Source: CAD feature listing. Evaluate the final solid. Frame: model axes, mm. A direction names the side the tool comes from. Give positions to 0.01 mm unless a question says otherwise; leave off trailing zeros. Order: outer loops, then holes, each group sorted by start corner. A loop starts at its lowest first (then second) coordinate and runs counter-clockwise, first axis right, second up. Notation, with made-up numbers: (70.25, 57) - (91.25, 57) arc R33 ccw to (91.25, 87) - close; hole circle Ø11 at (24, -32.5). An arc over 180 degrees is marked (long way). Use CSV: the item, a comma, the result in double quotes.
```python
from build123d import *
from build123d.topology import SkipClean

# Parameters (mm, degrees)
SKETCH1_3_W              = 17.39
SKETCH1_3_H              = 14
REVOLVE2_ANGLE           = 3
REVOLVE2_OTHER_WAY_ANGLE = 3
CIRPATTERN1_COUNT        = 6
CIRPATTERN1_ANGLE        = 25


with BuildPart() as part:
    # Sketch1 → Revolve1 (revolve)
    with BuildSketch(Plane.YZ, mode=Mode.PRIVATE) as revolve1_sk:
        Polygon((120, 13), (13, 13), (13, 4), (10, 4), (10, 3), (0, 3), (0, 0), (19, 0), (19, 10), (129, 10), (129, -5), (152.39, -5), (152.39, 5), (135, 5), (135, 19), (120, 19), align=None)
    revolve(revolve1_sk.sketch.rotate(Axis((0, 0, 0), (0, 0, 1)), 90), axis=Axis((0, 0, 0), (0, 0, 1)))

    # Sketch1<3> → Revolve2 (revolve)
    with BuildSketch(Plane.YZ):
        with Locations((143.695, 12)):
            Rectangle(SKETCH1_3_W, SKETCH1_3_H)
    revolve(axis=Axis((0, 0, 0), (0, 0, 1)), revolution_arc=REVOLVE2_ANGLE)

    # Sketch1<3> → Revolve2 other way (revolve)
    with SkipClean():  # the faces are left unmerged after this step: merging them gives an invalid solid
        with BuildSketch(Plane.YZ):
            with Locations((143.695, 12)):
                Rectangle(SKETCH1_3_W, SKETCH1_3_H)
        revolve(axis=Axis((0, 0, 0), (0, 0, -1)), revolution_arc=REVOLVE2_OTHER_WAY_ANGLE)
    add(part.part.scale(1), mode=Mode.REPLACE)  # the faces are merged on a copy

    # Sketch2 → Cut-Revolve4 (revolve, cut)
    with BuildSketch(Plane(origin=(0, 0, 8), x_dir=(0, 1, 0), z_dir=(0, 0, 1)), mode=Mode.PRIVATE) as cut_revolve4_sk:
        Polygon((111.823962377, 11.376893011), (151.671750301, 14.863122721), (151.810110042, 13.281663637), (111.962322119, 9.795433927), align=None)
    cut_revolve4 = revolve(cut_revolve4_sk.sketch.rotate(Axis((-9.795433927, 111.962322119, 8), (-0.08715574274765829, 0.9961946980917455, 0)), 180), axis=Axis((-9.795433927, 111.962322119, 8), (-0.08715574274765829, 0.9961946980917455, 0)), mode=Mode.SUBTRACT)

    # CirPattern1: Cut-Revolve4 ×6 about axis
    cirpattern1_axis = Axis((0, 0, 0), (0, 0, 1))
    for i in range(1, CIRPATTERN1_COUNT):
        add(cut_revolve4.rotate(cirpattern1_axis, i * CIRPATTERN1_ANGLE / (CIRPATTERN1_COUNT - 1)), mode=Mode.SUBTRACT)


solid = part.part
```
Item 1: First-contact query: pin 1 (6 mm diameter, centred on y = -119, z = -1.5, fed in from +X); pin 2 (10 mm diameter, centred on x = -75, z = 7.5, fed in from +Y); pin 3 (16 mm diameter, centred on x = -4, y = 2, fed in from +Z). Flat tips, straight axial feed; report the tip coordinate or a pass-through.
Filled in:
pin 1,"stops at x = 98.83"
pin 2,"stops at y = 135.01"
pin 3,"stops at z = 4"
Item 2: Mould query, pull axis X, two halves, no side actions, for faces 5 (the flat face through (-7.514, 143.377, 12.098)), 6 (the cylindrical face through (4.119, 18.548, 5.07)), 7 (the flat face through (1, -136, 5)). Classes: released by +X, released by -X, zero draft, split by the parting line, or undercut.
Filled in:
face 5,"released by -X"
face 6,"undercut"
face 7,"zero draft"
Item 3: Material intervals for line 1 (Y direction, x = 0, z = 3.6); line 2 (Y direction, x = 0, z = 5.25); line 3 (Y direction, x = 0, z = 10.5), sorted ascending. Write a range as from..to.
Filled in:
line 1,"y = -152.39..-129, -19..-10, 10..19, 129..152.39"
line 2,"y = -135..-129, -19..-13, 13..19, 129..152.39"
line 3,"y = -135..-13, 13..152.39"
Item 4: Section B-B on x = -113. Return the cut outline in (y, z), then the cut area to 3 significant figures.
Filled in:
outline,"(-102.24, -5) - (-62.23, -5) - (-62.23, 10) - (62.23, 10) - (62.23, -5) - (102.24, -5) - (102.24, 5) - (73.86, 5) - (73.86, 19) - (40.39, 19) - (40.39, 13) - (-40.39, 13) - (-40.39, 19) - (-73.86, 19) - (-73.86, 5) - (-102.24, 5) - close"
area,"1,760 mm2"
Item 5: Section A-A on y = -30.5. Return the cut outline in (x, z), then the cut area to 3 significant figures.
Filled in:
outline,"(-149.31, -5) - (-125.34, -5) - (-125.34, 10) - (125.34, 10) - (125.34, -5) - (149.31, -5) - (149.31, 5) - (131.51, 5) - (131.51, 19) - (116.06, 19) - (116.06, 13) - (-116.06, 13) - (-116.06, 19) - (-131.51, 19) - (-131.51, 5) - (-149.31, 5) - close"
area,"1,520 mm2"
Item 6: Set-up query: faces 1 (the cylindrical face through (10.316, 7.91, 8.437)), 2 (the flat face through (7.514, 143.377, 12.098)), 3 (the flat face through (-125, -35, -5)), 4 (the cylindrical face through (-123.043, -38.748, 2.395)). Return all of +Z, -Z, +X, -X, +Y, -Y with unobstructed straight access to the full face (end or side cutting, diameter ignored); none if empty.
Filled in:
face 1,"+Z"
face 2,"+Z, +X"
face 3,"-Z, +X, -X, +Y, -Y"
face 4,"-Z"
